Check sheet for the modelled part. Datum: model origin and axes. Units: mm. Give positions to 0.01 mm unless a question says otherwise; leave off trailing zeros. Loops run counter-clockwise (first coordinate to the right, second up) from the corner with the lowest first, then second, coordinate; pieces in that order, holes last. Notation, with made-up numbers: (-35, 35) -> (19, 35) arc R19 ccw to (19, 45) -> close; hole circle Ø5 at (-29.75, -32). An arc over 180 degrees is marked (long way). Write each question's results on one line, items separated by ' | '. Start each with the question number.
Item 1: Cross-section at B-B on y = 25. Enter the section's corners in (x, z).
Item 2: Cross-section at A-A on x = 135.5. Enter the section's corners in (y, z).
Item 3: Cross-section at D-D on z = 2.2. State how many separate pieces and enclosed holes the cut face has, then the cut area to 3 significant figures.
Item 4: Scan lines: line 1 along Y through (x, z) = (84.5, 2.25); line 2 along X through (y, z) = (131, 2.6); line 3 along X through (y, z) = (95, 1.85). Record each from-to range of solid material in increasing order.
Item 5: Gauge pin test, flat end, axial feed: pin 1 Ø0.9 at (y, z) = (35.5, 2) entering from +X. Record the tip position at first contact, or that the pin passes through.
Item 6: Cross-section at C-C on x = 88. Enter the section's corners in (y, z), then the cut area to 3 significant figures.
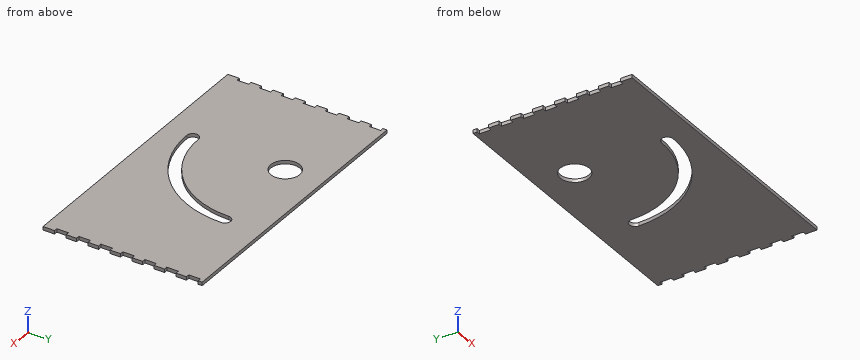
from build123d import *

# Parameters (mm, degrees)
SKETCH1_R           = 12.5
BOSS_EXTRUDE1_DEPTH = 3


with BuildPart() as part:
    # Sketch1 → Boss-Extrude1 (new body)
    with BuildSketch(Plane.XY):
        Polygon((244.5, 137.5), (244.5, 134), (241.5, 134), (241.5, 124), (244.5, 124), (244.5, 115), (241.5, 115), (241.5, 105), (244.5, 105), (244.5, 96), (241.5, 96), (241.5, 86), (244.5, 86), (244.5, 77), (241.5, 77), (241.5, 67), (244.5, 67), (244.5, 58), (241.5, 58), (241.5, 48), (244.5, 48), (244.5, 39), (241.5, 39), (241.5, 29), (244.5, 29), (244.5, 20), (241.5, 20), (241.5, 10), (244.5, 10), (244.5, 0), (-0.5, 0), (-0.5, 10), (2.5, 10), (2.5, 20), (-0.5, 20), (-0.5, 29), (2.5, 29), (2.5, 39), (-0.5, 39), (-0.5, 48), (2.5, 48), (2.5, 58), (-0.5, 58), (-0.5, 67), (2.5, 67), (2.5, 77), (-0.5, 77), (-0.5, 86), (2.5, 86), (2.5, 96), (-0.5, 96), (-0.5, 105), (2.5, 105), (2.5, 115), (-0.5, 115), (-0.5, 124), (2.5, 124), (2.5, 134), (-0.5, 134), (-0.5, 137.5), align=None)
        with Locations((84.5, 105)):
            Circle(SKETCH1_R, mode=Mode.SUBTRACT)
        with BuildLine():
            ThreePointArc((169.5, 105), (164.5, 110), (159.5, 105))
            ThreePointArc((159.5, 105), (137.533008589, 51.966991411), (84.5, 30))
            ThreePointArc((84.5, 30), (79.5, 25), (84.5, 20))
            ThreePointArc((84.5, 20), (144.604076401, 44.895923599), (169.5, 105))
        make_face(mode=Mode.SUBTRACT)
    extrude(amount=BOSS_EXTRUDE1_DEPTH)


solid = part.part
Answer sheet:
1) outline: (-0.5, 0) -> (79.5, 0) -> (79.5, 3) -> (-0.5, 3) -> close; (113.22, 0) -> (244.5, 0) -> (244.5, 3) -> (113.22, 3) -> close
2) outline: (0, 0) -> (37, 0) -> (37, 3) -> (0, 3) -> close; (50.01, 0) -> (137.5, 0) -> (137.5, 3) -> (50.01, 3) -> close
3) separate pieces: 1 | enclosed holes: 2 | area: 31,400 mm²
4) line 1: y = 0 to 20, 30 to 92.5, 117.5 to 137.5 | line 2: x = 2.5 to 241.5 | line 3: x = 2.5 to 77, 92 to 158.83, 168.91 to 241.5
5) pin 1: stops at x = 241.5
6) outline: (0, 0) -> (20.07, 0) -> (20.07, 3) -> (0, 3) -> close; (30.08, 0) -> (93, 0) -> (93, 3) -> (30.08, 3) -> close; (117, 0) -> (137.5, 0) -> (137.5, 3) -> (117, 3) -> close | area: 310 mm²
